from build123d import *

# Parameters (mm, degrees)
BOSS_EXTRUDE1_DEPTH            = 20
SKETCH3_R                      = 2.1
CUT_EXTRUDE1_DEPTH             = 66.357956669
F_4_2_4_2_DIAMETER_HOLE1_D     = 4.2
F_4_2_4_2_DIAMETER_HOLE1_DEPTH = 6
F_4_2_4_2_DIAMETER_HOLE1_TIP   = 1.2618073
F_4_2_4_2_DIAMETER_HOLE4_D     = 4.2
F_4_2_4_2_DIAMETER_HOLE4_DEPTH = 6
F_4_2_4_2_DIAMETER_HOLE4_TIP   = 1.2618073
FILLET2_R                      = 5


with BuildPart() as part:
    # Sketch1 → Boss-Extrude1 (new body)
    with BuildSketch(Plane(origin=(0, 0, 0), x_dir=(1, 0, 0), z_dir=(0, 1, 0))):
        with BuildLine():
            Line((28.15, -42.55), (45.4, -42.55))
            Line((45.4, -42.55), (45.4, 42.55))
            Line((45.4, 42.55), (-45.4, 42.55))
            Line((-45.4, 42.55), (-45.4, -42.55))
            Line((-45.4, -42.55), (-28.15, -42.55))
            Line((-28.15, -42.55), (-28.15, -33.579320378))
            ThreePointArc((-28.15, -33.579320378), (0, 23.55), (28.15, -33.579320378))
            Line((28.15, -33.579320378), (28.15, -42.55))
        make_face()
    extrude(amount=BOSS_EXTRUDE1_DEPTH)

    # Sketch3 → Cut-Extrude1 (cut, through all)
    with BuildSketch(Plane(origin=(0, 20, 0), x_dir=(1, 0, 0), z_dir=(0, 1, 0))):
        with Locations(Location((-30, 32.25, 0), (0, 0, 270))):
            Circle(SKETCH3_R)
        with Locations(Location((-20, 32.25, 0), (0, 0, 270))):
            Circle(SKETCH3_R)
        with Locations(Location((20, 32.25, 0), (0, 0, 90))):
            Circle(SKETCH3_R)
        with Locations(Location((30, 32.25, 0), (0, 0, 90))):
            Circle(SKETCH3_R)
    extrude(amount=-CUT_EXTRUDE1_DEPTH, mode=Mode.SUBTRACT)

    # Ø4.2 (4.2) Diameter Hole1
    with Locations(Plane(origin=(0, 0, -42.55), x_dir=(-1, 0, 0), z_dir=(0, 0, -1))):
        with Locations((-30, 10), (-10, 10), (10, 10), (30, 10)):
            Hole(F_4_2_4_2_DIAMETER_HOLE1_D / 2, depth=F_4_2_4_2_DIAMETER_HOLE1_DEPTH)
            with Locations((0, 0, -(F_4_2_4_2_DIAMETER_HOLE1_DEPTH + F_4_2_4_2_DIAMETER_HOLE1_TIP / 2))):  # 118° drill point
                Cone(0, F_4_2_4_2_DIAMETER_HOLE1_D / 2, F_4_2_4_2_DIAMETER_HOLE1_TIP, mode=Mode.SUBTRACT)

    # Ø4.2 (4.2) Diameter Hole4
    with Locations(Plane.ZY.offset(45.4)):
        with Locations((-17.45, 10), (22.55, 10)):
            Hole(F_4_2_4_2_DIAMETER_HOLE4_D / 2, depth=F_4_2_4_2_DIAMETER_HOLE4_DEPTH)
            with Locations((0, 0, -(F_4_2_4_2_DIAMETER_HOLE4_DEPTH + F_4_2_4_2_DIAMETER_HOLE4_TIP / 2))):  # 118° drill point
                Cone(0, F_4_2_4_2_DIAMETER_HOLE4_D / 2, F_4_2_4_2_DIAMETER_HOLE4_TIP, mode=Mode.SUBTRACT)

    # Sketch20 → Ø4.2 (4.2) Diameter Hole6 (revolve, cut)
    with BuildSketch(Plane(origin=(-37, 10, 42.55), x_dir=(0, -1, 0), z_dir=(1, 0, 0))):
        Polygon((0, 0), (0, 7.2618073), (2.1, 6), (2.1, 0), align=None)
    f_4_2_4_2_diameter_hole6 = revolve(axis=Axis((-37, 10, 48.9), (0, 0, -1)), mode=Mode.SUBTRACT)

    # Mirror2: Ø4.2 (4.2) Diameter Hole6 across plane
    add(f_4_2_4_2_diameter_hole6.mirror(Plane(origin=(0, 0, 0), x_dir=(0, 0, 1), z_dir=(1, 0, 0))), mode=Mode.SUBTRACT)

    # Fillet2
    fillet2_edges = [part.edges().sort_by_distance(p)[0] for p in [
        (28.15, 10, 33.579320378),
        (-28.15, 10, 33.579320378),
        (-45.4, 10, -42.55),
        (45.4, 10, -42.55),
    ]]
    fillet(fillet2_edges, radius=FILLET2_R)


solid = part.part
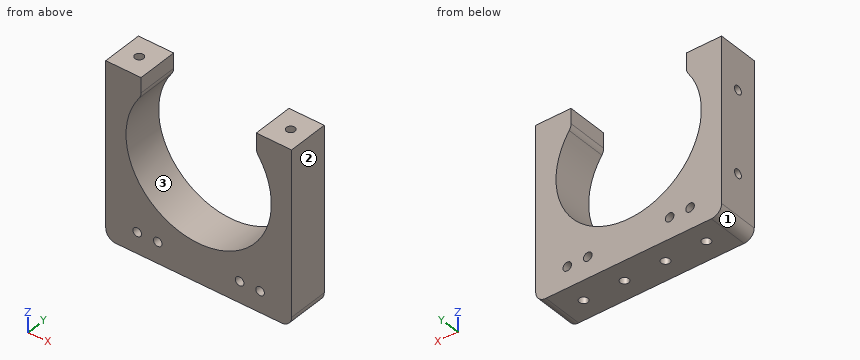
Can you work these out from the model? Positions are in its coordinate system, mm. Face numbers are marked on the shaded views. Round coordinates to 2 decimals unless told otherwise and drop trailing zeros. Loops run counter-clockwise (first coordinate to the right, second up) from the corner with the lowest first, then second, coordinate; pieces in that order, holes last. Notation, with made-up numbers: (70.5, -34) - (95.5, -34) arc R14 cw to (95.5, -16) - close; hole circle Ø2 at (68.5, 8). An arc over 180 degrees is marked (long way). Answer in a Markdown table with one row per item. Add a question column.
Q1. I need wall thicknesses on L1, parallel to Z at x = -40.85, y = 10; L2, parallel to X at y = 10, z = 37.5; L3, parallel to X at y = 6.75, z = -32.25. Which ranges of each line are inside material? Lowest first, please.
Q2. I want a section at B-B on y = 4. List the corners of the cut face in (x, z) for me.
Q3. I want a section at D-D on z = -9.5. List the corners of the cut face in (x, y) for me.
Q4. For pin 1 Ø4 at (x, z) = (-20, -32.25) entering from -Y; pin 2 Ø5.5 at (x, y) = (10, 10) entering from +Z; pin 3 Ø5.5 at (x, y) = (37, 10) entering from +Z; pin 4 Ø4 at (x, y) = (1, 3.5) entering from +Z, each with a flat end and sliding along its axis, tell me the tip position at first contact or that it passes through.
Q5. I want a section at C-C on x = -20. List the corners of the cut face in (y, z) for me.
Q6. I want a section at A-A on z = -32.25. List the corners of the cut face in (x, y) for me.
Q7. We'd pull the mould along Z, two halves only. Please class the marked faces 1, 2 and 3: pulls with the +Z half, pulls with the -Z half, needs draft (parallel to the pull), parting line crosses it, or undercut.
A:
| question | item | result |
|---|---|---|
| 1 | L1 | -42.53 to -19.55, -15.35 to 20.45, 24.65 to 42.55 |
| 1 | L2 | -45.4 to -39.1, -34.9 to -28.15, 28.15 to 34.9, 39.1 to 45.4 |
| 1 | L3 | -45.4 to -32.1, -27.9 to -22.1, -17.9 to 17.9, 22.1 to 27.9, 32.1 to 45.4 |
| 2 | outline | (-45.4, -37.55) arc R5 ccw to (-40.4, -42.55) - (40.4, -42.55) arc R5 ccw to (45.4, -37.55) - (45.4, 42.55) - (28.15, 42.55) - (28.15, 35.22) arc R5 ccw to (29.06, 32.34) arc R35.5 cw (long way) to (-29.06, 32.34) arc R5 ccw to (-28.15, 35.22) - (-28.15, 42.55) - (-45.4, 42.55) - close; hole circle Ø4.2 at (-30, -32.25); hole circle Ø4.2 at (-20, -32.25); hole circle Ø4.2 at (20, -32.25); hole circle Ø4.2 at (30, -32.25) |
| 3 | outline | (-45.4, 0) - (-28.29, 0) - (-28.29, 20) - (-45.4, 20) - close; (28.29, 0) - (45.4, 0) - (45.4, 20) - (28.29, 20) - close |
| 4 | pin 1 | through |
| 4 | pin 2 | z = -21.18 |
| 4 | pin 3 | z = 42.55 |
| 4 | pin 4 | z = -23.42 |
| 5 | outline | (0, -42.55) - (20, -42.55) - (20, -34.35) - (0, -34.35) - close; (0, -30.15) - (20, -30.15) - (20, -17.38) - (0, -17.38) - close |
| 6 | outline | (-45.4, 0) - (-32.1, 0) - (-32.1, 20) - (-45.4, 20) - close; (-27.9, 0) - (-22.1, 0) - (-22.1, 20) - (-27.9, 20) - close; (-17.9, 0) - (17.9, 0) - (17.9, 20) - (-17.9, 20) - close; (22.1, 0) - (27.9, 0) - (27.9, 20) - (22.1, 20) - close; (32.1, 0) - (45.4, 0) - (45.4, 20) - (32.1, 20) - close |
| 7 | face 1 | pulls with the -Z half |
| 7 | face 2 | needs draft |
| 7 | face 3 | undercut |
